Work out the finished part from the listing and answer in its coordinate system (mm). A direction names the side the tool comes from. Give positions to 0.01 mm unless a question says otherwise; leave off trailing zeros. Loops run counter-clockwise (first coordinate to the right, second up) from the corner with the lowest first, then second, coordinate; pieces in that order, holes last. Notation, with made-up numbers: (-28.5, 11.5) - (-7.5, 11.5) arc R17 ccw to (-7.5, 33.5) - close; hole circle Ø3 at (33.5, 81). An arc over 180 degrees is marked (long way). One line per item, written item: value.
Autodesk Inventor part; units mm, degrees
ref_plane "YZ Plane" through (0, 0, 0) normal (1, 0, 0) x (0, 1, 0)
ref_plane "XZ Plane" through (0, 0, 0) normal (0, 1, 0) x (-1, 0, 0)
ref_plane "XY Plane" through (0, 0, 0) normal (0, 0, 1) x (1, 0, 0)
sketch "Sketch1" plane through (0, 0, 0) normal (0, 0, 1) x (1, 0, 0)
  circle A0 centre (0, 0) radius 12.7
  line L0 (12.7, 0) -> (12.7, 38.1)
  line L1 (-12.7, 0) -> (-12.7, 38.1)
  line L2 (-12.7, 38.1) -> (12.7, 38.1)
  circle A1 centre (0, 0) radius 3.175
  dimension "d0" = 25.4
  dimension "d1" = 38.1
  dimension "d3" = 6.35
extrude "Extrusion1" add sketch "Sketch1" along normal blind 3.175
sketch "Sketch2" plane through (0, 0, 3.175) normal (0, 0, 1) x (1, 0, 0)
  line L0 (12.7, 38.1) -> (-12.7, 38.1)
  line L1 (-12.7, 38.1) -> (12.7, 38.1)
  line L2 (12.7, 38.1) -> (12.7, 34.925)
  line L3 (12.7, 34.925) -> (-12.7, 34.925)
  line L4 (-12.7, 34.925) -> (-12.7, 38.1)
  point P0 (0, 0)
  dimension "d6" = 25.4
  dimension "d7" = 3.175
extrude "Extrusion2" add sketch "Sketch2" along normal blind 25.4
properties part number "Roller holder"
1. Flat-ended cylindrical pins translate along their axes: pin 1 Ø5.5 at (x, y) = (0, 0) entering from -Z; pin 2 Ø7.5 at (x, y) = (4, 10) entering from +Z (3 decimals); pin 3 Ø10 at (x, z) = (9, 19.5) entering from -Y (3 decimals). Find the tip coordinate at first contact, or state that the pin passes through.
Output:
pin 1: passes through
pin 2: stops at z = 3.175
pin 3: stops at y = 34.925
2. For faces 4 (the flat face through (-12.7, 26, 3)), 5 (the flat face through (0, 11, 3.175)), determine the directions among +Z, -Z, +X, -X, +Y, -Y from which every point of the face is accessible in a straight line to the end or side of a thin tool.
Output:
face 4: +Z, -Z, -X, +Y, -Y
face 5: +Z, +X, -X, -Y
3. Section A-A (x = 0) is taken. Write down the section's boundary in (y, z) (3 decimals).
Output:
outline: (-12.7, 0) - (-3.175, 0) - (-3.175, 3.175) - (-12.7, 3.175) - close; (3.175, 0) - (38.1, 0) - (38.1, 28.575) - (34.925, 28.575) - (34.925, 3.175) - (3.175, 3.175) - close
4. Section B-B (y = -2) is taken. Write down the section's boundary in (x, z) (3 decimals).
Output:
outline: (-12.542, 0) - (-2.466, 0) - (-2.466, 3.175) - (-12.542, 3.175) - close; (2.466, 0) - (12.542, 0) - (12.542, 3.175) - (2.466, 3.175) - close
5. The mould has two halves that part along Y. Classify faces 1 (the flat face through (0, 34.925, 16)), 2 (the flat face through (0, 38.1, 14)), 3 (the cylindrical face through (-0.69, 3.1, 1.57)): released by +Y, released by -Y, zero draft, split by the parting line, or undercut.
Output:
face 1: released by -Y
face 2: released by +Y
face 3: undercut
6. Section D-D (x = -6.5) is taken. Write down the section's boundary in (y, z) (3 decimals), and give its area (3 significant figures).
Output:
outline: (-10.911, 0) - (38.1, 0) - (38.1, 28.575) - (34.925, 28.575) - (34.925, 3.175) - (-10.911, 3.175) - close
area: 236 mm²
7. Section C-C (z = 5) is taken. Write down the section's boundary in (x, y) (3 decimals), and give its area (3 significant figures).
Output:
outline: (-12.7, 34.925) - (12.7, 34.925) - (12.7, 38.1) - (-12.7, 38.1) - close
area: 80.6 mm²
8. Find the intervals of material crossed by line 1 along Y through (x, z) = (0, 2.45) (3 decimals); line 2 along Y through (x, z) = (9.75, 27.5) (3 decimals); line 3 along Z through (x, y) = (-10.5, 31) (3 decimals), in increasing order.
Output:
line 1: y = -12.7 to -3.175, 3.175 to 38.1
line 2: y = 34.925 to 38.1
line 3: z = 0 to 3.175
